```python
from build123d import *

# Parameters (mm, degrees)
F0_R     = 3.07975
F1_DEPTH = 6.35
F2_R     = 3.71475
F2_R_2   = 2.00025
F3_DEPTH = 3.175
F4_SIZE  = 1.27


# Not quite as in the source:
# - a feature names something its author has since deleted; it is built from what else it names


with BuildPart() as f1:
    # F0 (on Top) → F1 (new body)
    with BuildSketch(Plane.XY):
        with BuildLine():
            ThreePointArc((-4.445, 0), (-4.106644522, 1.7010278569), (-3.1430896424, 3.1430896424))
            Line((-3.1430896424, 3.1430896424), (-7.1842048969, 7.1842048969))
            ThreePointArc((-7.1842048969, 7.1842048969), (-9.3866160503, 3.8880636728), (-10.16, 0))
            ThreePointArc((-10.16, 0), (-9.3866160503, -3.8880636728), (-7.1842048969, -7.1842048969))
            Line((-7.1842048969, -7.1842048969), (-3.1430896424, -3.1430896424))
            ThreePointArc((-3.1430896424, -3.1430896424), (-4.106644522, -1.7010278569), (-4.445, 0))
        make_face()
        with BuildLine():
            ThreePointArc((3.1430896424, -3.1430896424), (4.106644522, -1.7010278569), (4.445, 0))
            ThreePointArc((4.445, 0), (4.106644522, 1.7010278569), (3.1430896424, 3.1430896424))
            ThreePointArc((3.1430896424, 3.1430896424), (0, 4.445), (-3.1430896424, 3.1430896424))
            ThreePointArc((-3.1430896424, 3.1430896424), (-4.106644522, 1.7010278569), (-4.445, 0))
            ThreePointArc((-4.445, 0), (-4.106644522, -1.7010278569), (-3.1430896424, -3.1430896424))
            ThreePointArc((-3.1430896424, -3.1430896424), (0, -4.445), (3.1430896424, -3.1430896424))
        make_face()
        Circle(F0_R, mode=Mode.SUBTRACT)
        with BuildLine():
            ThreePointArc((3.1430896424, 3.1430896424), (4.106644522, 1.7010278569), (4.445, 0))
            ThreePointArc((4.445, 0), (4.106644522, -1.7010278569), (3.1430896424, -3.1430896424))
            Line((3.1430896424, -3.1430896424), (7.1842048969, -7.1842048969))
            ThreePointArc((7.1842048969, -7.1842048969), (9.3866160503, -3.8880636728), (10.16, 0))
            ThreePointArc((10.16, 0), (9.3866160503, 3.8880636728), (7.1842048969, 7.1842048969))
            Line((7.1842048969, 7.1842048969), (3.1430896424, 3.1430896424))
        make_face()
        Circle(F0_R)
    extrude(amount=F1_DEPTH)

    # F2 (on face) → F3 (cut)
    with BuildSketch(Plane.XY.offset(6.35)):
        with BuildLine():
            ThreePointArc((6.298995158, -1.36525), (6.4085819845, -0.6865307789), (6.44525, 0))
            ThreePointArc((6.44525, 0), (6.4085819845, 0.6865307789), (6.298995158, 1.36525))
            ThreePointArc((6.298995158, 1.36525), (5.658033773, 3.0867298855), (4.5574799814, 4.5574799814))
            Line((4.5574799814, 4.5574799814), (3.1430896424, 3.1430896424))
            ThreePointArc((3.1430896424, 3.1430896424), (0, 4.445), (-3.1430896424, 3.1430896424))
            Line((-3.1430896424, 3.1430896424), (-4.5574799814, 4.5574799814))
            ThreePointArc((-4.5574799814, 4.5574799814), (-5.658033773, 3.0867298855), (-6.298995158, 1.36525))
            ThreePointArc((-6.298995158, 1.36525), (-6.44525, 0), (-6.298995158, -1.36525))
            ThreePointArc((-6.298995158, -1.36525), (-5.658033773, -3.0867298855), (-4.5574799814, -4.5574799814))
            Line((-4.5574799814, -4.5574799814), (-3.1430896424, -3.1430896424))
            ThreePointArc((-3.1430896424, -3.1430896424), (0, -4.445), (3.1430896424, -3.1430896424))
            Line((3.1430896424, -3.1430896424), (4.5574799814, -4.5574799814))
            ThreePointArc((4.5574799814, -4.5574799814), (5.658033773, -3.0867298855), (6.298995158, -1.36525))
        make_face()
        Circle(F2_R, mode=Mode.SUBTRACT)
        with BuildLine():
            ThreePointArc((6.298995158, 1.36525), (6.4085819845, 0.6865307789), (6.44525, 0))
            ThreePointArc((6.44525, 0), (6.4085819845, -0.6865307789), (6.298995158, -1.36525))
            Line((6.298995158, -1.36525), (10.0678544108, -1.36525))
            ThreePointArc((10.0678544108, -1.36525), (10.16, 0), (10.0678544108, 1.36525))
            Line((10.0678544108, 1.36525), (6.298995158, 1.36525))
        make_face()
        with BuildLine():
            ThreePointArc((-6.298995158, -1.36525), (-6.44525, 0), (-6.298995158, 1.36525))
            Line((-6.298995158, 1.36525), (-10.0678544108, 1.36525))
            ThreePointArc((-10.0678544108, 1.36525), (-10.16, 0), (-10.0678544108, -1.36525))
            Line((-10.0678544108, -1.36525), (-6.298995158, -1.36525))
        make_face()
        Circle(F2_R_2)
    extrude(amount=-F3_DEPTH, mode=Mode.SUBTRACT)

    # F4
    f4_edges = [f1.edges().sort_by_distance(p)[0] for p in [
        (-2.00025, 0, 3.175),
    ]]
    chamfer(f4_edges, length=F4_SIZE)


solid = f1.part
```
CAD build for the part. Positions are in the model's coordinates, mm. A direction names the side the tool comes from. Round coordinates to 2 decimals unless told otherwise and drop trailing zeros. Loops run counter-clockwise (first coordinate to the right, second up) from the corner with the lowest first, then second, coordinate; pieces in that order, holes last. Notation, with made-up numbers: M 49,-0.5 L 80,-0.5 A32 cw 80,28.5 Z; hole C 9,-14.5 d4. An arc over 180 degrees is marked long. Return JSON: item names as keys, results as strings. Group by question number.
(1) Saw through at C-C, the plane y = -6.5. List the corners of the cut face in (x, z).
(2) Saw through at D-D, the plane x = 8. List the corners of the cut face in (y, z) (3 decimals).
(3) Saw through at A-A, the plane z = 5. List the corners of the cut face in (x, y).
(4) Tool access for faces 1 (the flat face through (-8, -1.365, 5)), 2 (the flat face through (-6, 6, 3)), 3 (the flat face through (8, 1.365, 5)), 4 (the cylindrical face through (-5.646, 3.109, 4.785)), 5 (the flat face through (-6, -6, 3)): list every direction of +Z, -Z, +X, -X, +Y, -Y with a clear straight run to the whole face (end or side of a thin tool).
(5) Mould opens along Y. For faces 6 (the cylindrical face through (-0.805, -3.626, 4.785)), 7 (the flat face through (-8, 1.365, 5)), 8 (the flat face through (6, 6, 3)) say: +Y half, -Y half, draft (parallel to the pull), parting line (faces both ways), or undercut.
(6) Wall check: probe 1 along X at (y, z) = (3, 3.25); probe 2 along Y at (x, z) = (0, 5.2); probe 3 along X at (y, z) = (3.5, 1.75). Give the ranges that are in metal, low to high. Write a range as [from, to].
(7) Drop flat-ended pins along their axis: P1, Ø0.7, axis at x = 0, y = 0, coming from the +Z side (3 decimals); P2, Ø8, axis at x = -3, y = -4.5, coming from the +Z side; P3, Ø3, axis at y = -5, z = 3, coming from the +X side; P4, Ø2.5, axis at x = -8.5, z = 5.5, coming from the -Y side. Give the stop position or say it passes through.
(8) Saw through at B-B, the plane z = 2. List the corners of the cut face in (x, y) (3 decimals).
Answer list:
{
 "1": {"outline": "M -7.81,0 L -6.5,0 L -6.5,6.35 L -7.81,6.35 Z; M 6.5,0 L 7.81,0 L 7.81,6.35 L 6.5,6.35 Z"},
 "2": {"outline": "M -6.263,0 L 6.263,0 L 6.263,6.35 L 1.365,6.35 L 1.365,3.175 L -1.365,3.175 L -1.365,6.35 L -6.263,6.35 Z"},
 "3": {"outline": "M -10.07,-1.37 A10.16 ccw -7.18,-7.18 L -4.56,-4.56 A6.45 cw -6.3,-1.37 Z; M -10.07,1.37 L -6.3,1.37 A6.45 cw -4.56,4.56 L -7.18,7.18 A10.16 ccw Z; C 0,0 d7.43; M 4.56,-4.56 L 7.18,-7.18 A10.16 ccw 10.07,-1.37 L 6.3,-1.37 A6.45 cw Z; M 4.56,4.56 A6.45 cw 6.3,1.37 L 10.07,1.37 A10.16 ccw 7.18,7.18 Z; hole C 0,0 d4"},
 "4": {"face 1": "+Z, -X", "face 2": "+Z, -Z, +Y", "face 3": "+Z, +X", "face 4": "+Z", "face 5": "+Z, -Z, -Y"},
 "5": {"face 6": "parting line", "face 7": "undercut", "face 8": "+Y half"},
 "6": {"probe 1": "[-9.71, -5.7], [-2.19, 2.19], [5.7, 9.71]", "probe 2": "[-3.71, -2], [2, 3.71]", "probe 3": "[-9.54, -3.5], [-2.74, 2.74], [3.5, 9.54]"},
 "7": {"P1": "z = 3.175", "P2": "z = 6.35", "P3": "x = 9.54", "P4": "y = -7.12"},
 "8": {"outline": "M -7.184,-7.184 L -3.143,-3.143 A4.445 ccw 3.143,-3.143 L 7.184,-7.184 A10.16 ccw 7.184,7.184 L 3.143,3.143 A4.445 ccw -3.143,3.143 L -7.184,7.184 A10.16 ccw Z"}
}
